Work out the finished part from the listing and answer in its coordinate system (mm). A direction names the side the tool comes from. Round coordinates to 2 decimals unless told otherwise and drop trailing zeros. Order: outer loops, then holes, each group sorted by start corner. A loop starts at its lowest first (then second) coordinate and runs counter-clockwise, first axis right, second up. Notation, with made-up numbers: (-31.75, -3) -> (1.25, -3) arc R27 cw to (1.25, 31) -> close; hole circle Ø1 at (8, 75). An arc over 180 degrees is marked (long way). Use one line per item in the form item = value.
```python
from build123d import *

# Parameters (mm, degrees)
F1_DEPTH = 568.325
F2_W     = 9.525
F2_H     = 9.525
F3_DEPTH = 50.8
F4_R     = 6.35


with BuildPart() as f1:
    # F0 (on Right) → F1 (new body)
    with BuildSketch(Plane.YZ):
        Polygon((0, 50.8), (0, 0), (9.525, 0), (9.525, 9.525), (19.05, 9.525), (19.05, 0), (28.575, 0), (28.575, 50.8), align=None)
    extrude(amount=F1_DEPTH)

    # F2 (on face) → F3 (cut)
    with BuildSketch(Plane.XY.offset(50.8)):
        with Locations((4.7625, 23.8125)):
            Rectangle(F2_W, F2_H)
        with Locations((4.7625, 4.7625)):
            Rectangle(F2_W, F2_H)
        with Locations((563.5625, 23.8125)):
            Rectangle(F2_W, F2_H)
        with Locations((563.5625, 4.7625)):
            Rectangle(F2_W, F2_H)
    extrude(amount=-F3_DEPTH, mode=Mode.SUBTRACT)

    # F4
    f4_edges = [f1.edges().sort_by_distance(p)[0] for p in [
        (284.1625, 0, 50.8),
        (284.1625, 28.575, 50.8),
    ]]
    fillet(f4_edges, radius=F4_R)


solid = f1.part
```
Item 1: For faces 4 (the flat face through (563, 9.525, 30)), 5 (the flat face through (558.8, 24, 26)), 6 (the flat face through (9.525, 5, 26)), 7 (the flat face through (9.525, 24, 26)), determine the directions among +Z, -Z, +X, -X, +Y, -Y from which every point of the face is accessible in a straight line to the end or side of a thin tool.
Findings:
face_4 = +Z, -Z, +X, -Y
face_5 = +Z, -Z, +X, +Y
face_6 = +Z, -Z, -X, -Y
face_7 = +Z, -Z, -X, +Y
Item 2: The part is cut by section A-A, the plane x = 271. Give the vertices of the cut face in (y, z) (3 decimals), and give its area (3 significant figures).
Findings:
outline = (0, 0) -> (9.525, 0) -> (9.525, 9.525) -> (19.05, 9.525) -> (19.05, 0) -> (28.575, 0) -> (28.575, 44.45) arc R6.35 ccw to (22.225, 50.8) -> (6.35, 50.8) arc R6.35 ccw to (0, 44.45) -> close
area = 1,340 mm^2
Item 3: Flat-ended cylindrical pins translate along their axes: P1, Ø5, axis at x = 563, z = 22.5, coming from the -Y side (3 decimals); P2, Ø6, axis at y = 23, z = 23.5, coming from the +X side; P3, Ø3, axis at x = 562, z = 20.5, coming from the +Y side. Find the tip coordinate at first contact, or state that the pin passes through.
Findings:
P1 = 9.525
P2 = 558.8
P3 = 19.05
Item 4: Consider line 1 along Y through (x, z) = (26, 6) (3 decimals); line 2 along X through (y, z) = (5.5, 22) (3 decimals); line 3 along Z through (x, y) = (440, 17) (3 decimals). Determine where each line is inside the solid, lowest interval first.
Findings:
line_1 = 0 to 9.525, 19.05 to 28.575
line_2 = 9.525 to 558.8
line_3 = 9.525 to 50.8
Item 5: Determine the mould class of faces 1 (the flat face through (280, 0, 23)), 2 (the flat face through (280, 14, 9.525)), 3 (the flat face through (5, 19.05, 30)) for opening direction Y: released by +Y, released by -Y, zero draft, split by the parting line, or undercut.
Findings:
face_1 = released by -Y
face_2 = undercut
face_3 = released by +Y
Item 6: The part is cut by section B-B, the plane z = 33. Give the vertices of the cut face in (x, y) (3 decimals).
Findings:
outline = (0, 9.525) -> (9.525, 9.525) -> (9.525, 0) -> (558.8, 0) -> (558.8, 9.525) -> (568.325, 9.525) -> (568.325, 19.05) -> (558.8, 19.05) -> (558.8, 28.575) -> (9.525, 28.575) -> (9.525, 19.05) -> (0, 19.05) -> close
